Source: CAD feature listing. Evaluate the final solid. Frame: model axes, mm. Give positions to 0.01 mm unless a question says otherwise; leave off trailing zeros. Order: outer loops, then holes, each group sorted by start corner. A loop starts at its lowest first (then second) coordinate and runs counter-clockwise, first axis right, second up.
from build123d import *

# Parameters (mm, degrees)
CHAMFER1_SIZE      = 0.2
CUT_EXTRUDE1_DEPTH = 0.75


with BuildPart() as part:
    # Sketch1 → Revolve1 (revolve)
    with BuildSketch(Plane.XY):
        Polygon((0, 1), (-1, 2), (-1.2, 2), (-1.2, 0), (8.8, 0), (8.8, 1), align=None)
    revolve(axis=Axis((-1.2, 0, 0), (1, 0, 0)))

    # Chamfer1
    chamfer1_edges = [part.edges().sort_by_distance(p)[0] for p in [
        (8.8, -1, 0),
    ]]
    chamfer(chamfer1_edges, length=CHAMFER1_SIZE)

    # Sketch2 → Cut-Extrude1 (cut)
    with BuildSketch(Plane.ZY.offset(1.2)):
        Polygon((-0.75055535, 0), (-0.375277675, -0.65), (0.375277675, -0.65), (0.75055535, 0), (0.375277675, 0.65), (-0.375277675, 0.65), align=None)
    extrude(amount=-CUT_EXTRUDE1_DEPTH, mode=Mode.SUBTRACT)


solid = part.part
(1) Pin query (flat end, axial travel): pin 1 Ø0.7 at (y, z) = (0, -0.5) entering from -X; pin 2 Ø1.5 at (x, y) = (5.5, 0.5) entering from -Z; pin 3 Ø1 at (x, y) = (6, 0.5) entering from +Z; pin 4 Ø1.5 at (x, z) = (3.5, 0) entering from -Y. Return the tip coordinate at first contact, or that it passes through.
(2) Section B-B, the plane x = 3.25. Return loops of the section in (y, z).
(3) Draft query along Y for faces 1 (the flat face through (-1.2, 1, 0)), 2 (the flat face through (-0.45, 0, 0)), 3 (the cylindrical face through (4, 0, -1)). Return one class per face: +Y half, -Y half, draft (parallel to the pull), parting line (faces both ways), or undercut.
(4) Section A-A, the plane z = 0. Return loops of the section in (x, y), plus the area to 3 significant figures.
(5) Line query: line 1 along X through (y, z) = (0.35, -0.25); line 2 along Z through (x, y) = (-0.5, 0.6); line 3 along Y through (x, z) = (1, 0.2). Output: solid intervals per line, ascending.
Checks:
1. pin 1: stops at x = -1.2
1. pin 2: stops at z = -1
1. pin 3: stops at z = 1
1. pin 4: stops at y = -1
2. outline: circle Ø2 at (0, 0)
3. face 1: draft
3. face 2: undercut
3. face 3: parting line
4. outline: (-1.2, -2) - (-1, -2) - (0, -1) - (8.6, -1) - (8.8, -0.8) - (8.8, 0.8) - (8.6, 1) - (0, 1) - (-1, 2) - (-1.2, 2) - (-1.2, 0.65) - (-0.45, 0.65) - (-0.45, -0.65) - (-1.2, -0.65) - close
4. area: 20.4 mm2
5. line 1: x = -0.45 to 8.8
5. line 2: z = -1.37 to -0.4, 0.4 to 1.37
5. line 3: y = -0.98 to 0.98
